Geometry: final body of the model. Coordinates: model frame, mm. A direction names the side the tool comes from. Round coordinates to 2 decimals unless told otherwise and drop trailing zeros. Loops run counter-clockwise (first coordinate to the right, second up) from the corner with the lowest first, then second, coordinate; pieces in that order, holes last. Notation, with made-up numbers: (1, 74) - (21, 74) arc R20 ccw to (21, 108) - close; hole circle Ø2 at (88.5, 85.25). An arc over 180 degrees is marked (long way). Write item = value, one per line. Start each with the question number.
Item 1: Line query: line 1 (X direction, y = 0.3, z = 7.5); line 2 (Y direction, x = 0, z = 4); line 3 (X direction, y = -0.2, z = 7). Output: solid intervals per line, ascending. Write a range as from..to.
Item 2: Draft query along Y for faces 3 (the flat face through (0, -2.412, 6)), 4 (the cylindrical face through (1.3, -0.1, 9)), 5 (the flat face through (-0.4, -0.4, 0)), 6 (the cylindrical face through (0.58, -0.856, 2.958)). Return one class per face: pulls with the +Y half, pulls with the -Y half, needs draft (parallel to the pull), parting line crosses it, or undercut.
Item 3: Section A-A (x = 0.2). Return loops of the section in (y, z), plus the area to 3 significant figures.
Item 4: Section B-B (z = 8.25). Return loops of the section in (x, y), plus the area to 3 significant figures.
Item 5: Section C-C (y = 0.2). Return loops of the section in (x, z).
Item 6: Access query for faces 1 (the flat face through (-0.4, -1.3, 12)), 2 (the flat face through (0, -1, 6)). Directions: +Z, -Z, +X, -X, +Y, -Y. A direction counts if a zero-diameter tool reaches every point of the face in a straight line with its end or side. Return the directions, or none.
Item 7: Section D-D (x = 1.2). Return loops of the section in (y, z), plus the area to 3 significant figures.
from build123d import *

# Parameters (mm, degrees)
ESQUISSE1_W             = 6
ESQUISSE1_H             = 4
ESQUISSE1_R             = 0.5
BOSS_EXTRU_1_DEPTH      = 12
ESQUISSE2_R             = 1
ENL_V_MAT_EXTRU_1_DEPTH = 6


with BuildPart() as part:
    # Esquisse1 → Boss.-Extru.1 (new body)
    with BuildSketch(Plane.XY):
        with Locations((0.349498461, -0.412280702)):
            Rectangle(ESQUISSE1_W, ESQUISSE1_H)
        with Locations((0.349498461, -0.412280702)):
            Circle(ESQUISSE1_R, mode=Mode.SUBTRACT)
    extrude(amount=BOSS_EXTRU_1_DEPTH)

    # Esquisse2 → Enlèv. mat.-Extru.1 (cut)
    with BuildSketch(Plane.XY.offset(12)):
        with Locations((0.349498461, -0.412280702)):
            Circle(ESQUISSE2_R)
    extrude(amount=-ENL_V_MAT_EXTRU_1_DEPTH, mode=Mode.SUBTRACT)


solid = part.part
Taken from the geometry:
q1.line_1 = -2.65..-0.35, 1.05..3.35
q1.line_2 = -2.41..-0.77, -0.05..1.59
q1.line_3 = -2.65..-0.63, 1.33..3.35
q2.face_3 = pulls with the -Y half
q2.face_4 = undercut
q2.face_5 = needs draft
q2.face_6 = undercut
q3.outline = (-2.41, 0) - (-0.89, 0) - (-0.89, 6) - (-1.4, 6) - (-1.4, 12) - (-2.41, 12) - close; (0.06, 0) - (1.59, 0) - (1.59, 12) - (0.58, 12) - (0.58, 6) - (0.06, 6) - close
q3.area = 30.4 mm^2
q4.outline = (-2.65, -2.41) - (3.35, -2.41) - (3.35, 1.59) - (-2.65, 1.59) - close; hole circle Ø2 at (0.35, -0.41)
q4.area = 20.9 mm^2
q5.outline = (-2.65, 0) - (3.35, 0) - (3.35, 12) - (1.14, 12) - (1.14, 6) - (-0.44, 6) - (-0.44, 12) - (-2.65, 12) - close
q6.face_1 = +Z, +X, -X, +Y, -Y
q6.face_2 = +Z
q7.outline = (-2.41, 0) - (1.59, 0) - (1.59, 12) - (0.11, 12) - (0.11, 6) - (-0.94, 6) - (-0.94, 12) - (-2.41, 12) - close
q7.area = 41.7 mm^2
